Autodesk Inventor part; units mm, degrees
ref_plane "YZ Plane" through (0, 0, 0) normal (1, 0, 0) x (0, 1, 0)
ref_plane "XZ Plane" through (0, 0, 0) normal (0, 1, 0) x (-1, 0, 0)
ref_plane "XY Plane" through (0, 0, 0) normal (0, 0, 1) x (1, 0, 0)
ref_plane "Work Plane1" through (1.1136, 1.5, 0.2896) normal (0, -1, 0) x (1, 0, 0)
sketch "Sketch3" plane through (1.1136, 1.5, 0.2896) normal (0, -1, 0) x (1, 0, 0)
  line L0 (-8.5, 0) -> (-8.5, 5) construction
  line L1 (-8.5, 5) -> (-1.5, 5) construction
  line L2 (-1.5, 5) -> (-1.5, 0) construction
  line L3 (0, 0) -> (-1.5, 0) construction
  line L4 (0, 0) -> (0, 6) construction
  line L5 (0, 6) -> (-22.065, 6) construction
  line L6 (-22.065, 0) -> (-22.065, 6) construction
  line L7 (-20.565, 0) -> (-22.065, 0) construction
  line L8 (-20.565, 0) -> (-20.565, 5) construction
  line L9 (-20.565, 5) -> (-13.565, 5) construction
  line L10 (-13.565, 5) -> (-13.565, 0) construction
  line L11 (-8.5, 0) -> (-13.565, 0) construction
  line L12 (-0.8, 0) -> (-21.265, 0)
  line L13 (-21.265, 0) -> (-21.265, 5.3)
  line L14 (-21.265, 5.3) -> (-0.8, 5.3)
  line L15 (-0.8, 5.3) -> (-0.8, 0)
  point P0 (-1.1136, -0.2896)
  dimension "d26" = 0.8
  dimension "d27" = 0.8
  dimension "d28" = 0.7
extrude "Extrusion3" add sketch "Sketch3" along normal blind 3
sketch "Sketch4" plane through (1.1136, 1.5, 0.2896) normal (0, 1, 0) x (1, 0, 0)
  line L0 (-8.5, 0) -> (-8.5, -5) construction
  line L1 (-8.5, -5) -> (-1.5, -5) construction
  line L2 (-1.5, -5) -> (-1.5, 0) construction
  line L3 (0, 0) -> (-1.5, 0) construction
  line L4 (0, 0) -> (0, -6) construction
  line L5 (0, -6) -> (-22.065, -6) construction
  line L6 (-22.065, 0) -> (-22.065, -6) construction
  line L7 (-20.565, 0) -> (-22.065, 0) construction
  line L8 (-20.565, 0) -> (-20.565, -5) construction
  line L9 (-20.565, -5) -> (-13.565, -5) construction
  line L10 (-13.565, -5) -> (-13.565, 0) construction
  line L11 (-8.5, 0) -> (-13.565, 0) construction
  line L12 (-2, 0) -> (-8, 0)
  line L13 (-8, 0) -> (-8, -4.3)
  line L14 (-8, -4.3) -> (-2, -4.3)
  line L15 (-2, -4.3) -> (-2, 0)
  line L16 (-0.8, 0) -> (-21.265, 0)
  line L17 (-14.065, 0) -> (-20.065, 0)
  line L18 (-20.065, 0) -> (-20.065, -4.3)
  line L19 (-20.065, -4.3) -> (-14.065, -4.3)
  line L20 (-14.065, -4.3) -> (-14.065, 0)
  point P0 (-1.1136, 0.2896)
  point P1 (-5, 0)
  point P2 (-11.0325, 0)
  dimension "d31" = 0.5
  dimension "d32" = 0.5
  dimension "d33" = 0.7
  dimension "d34" = 0.7
  dimension "d35" = 0.5
  dimension "d36" = 0.5
extrude "Extrusion4" add sketch "Sketch4" along normal blind 7
fillet "Fillet6" radius 1 4 edges at (-20.1514, 0, 5.5896) (-20.1514, 0, 0.2896) (0.3136, 0, 5.5896) (0.3136, 0, 0.2896)
fillet "Fillet6" radius 1 4 edges at (-3.8864, 8.5, 4.5896) (-3.8864, 8.5, 0.2896) (-15.9514, 8.5, 0.2896) (-15.9514, 8.5, 4.5896)
properties part number "Holster_Button"
Source: CAD feature listing. Evaluate the final solid. Frame: model axes, mm. A direction names the side the tool comes from. Round coordinates to 2 decimals unless told otherwise and drop trailing zeros. Loops run counter-clockwise (first coordinate to the right, second up) from the corner with the lowest first, then second, coordinate; pieces in that order, holes last. Notation, with made-up numbers: M 81,-31 L 100,-31 A11 cw 100,-21 Z; hole C 13,66.5 d4. An arc over 180 degrees is marked long. Use a Markdown table: item, result. Add a question column.
1. Cut plane C-C, the plane x = -1.25. Output: boundary loops of the cut face in (y, z).
2. Set-up query: faces 1 (the flat face through (-0.886, 5, 2)), 2 (the flat face through (-12.951, 5, 2)), 3 (the flat face through (-16, 4, 4.59)). Return all of +Z, -Z, +X, -X, +Y, -Y with unobstructed straight access to the full face (end or side cutting, diameter ignored); none if empty.
3. Cut plane D-D, the plane z = 4.15. Output: boundary loops of the cut face in (x, y).
4. Cut plane B-B, the plane z = 3.3. Output: boundary loops of the cut face in (x, y), and give its area (3 significant figures).
5. Ray query, line 1 along X through (y, z) = (7.25, 2.7); line 2 along Y through (x, z) = (-18.25, 4.9); line 3 along Z through (x, y) = (-2.5, 3). Return the intervals inside material, ascending. Write a range as [from, to].
6. Contact query for flat-ended pins moving along their axis: pin 1 (2 mm diameter, centred on y = 4, z = 1.5, fed in from -X); pin 2 (1.8 mm diameter, centred on x = -15, y = 4.5, fed in from +Z); pin 3 (2 mm diameter, centred on y = 4.5, z = 1.5, fed in from +X). Output: stop coordinate, or through.
7. Cut plane A-A, the plane y = 4.5. Output: boundary loops of the cut face in (x, z).
Solution:
| question | item | result |
|---|---|---|
| 1 | outline | M -1.5,0.29 L 7.5,0.29 A1 ccw 8.5,1.29 L 8.5,3.59 A1 ccw 7.5,4.59 L 1.5,4.59 L 1.5,5.59 L -1.5,5.59 Z |
| 2 | face 1 | +Z, -Z, +X, +Y |
| 2 | face 2 | +Z, -Z, +Y |
| 2 | face 3 | +Z, +X, -X, +Y |
| 3 | outline | M -20.15,-1.5 L 0.31,-1.5 L 0.31,1.5 L -0.89,1.5 L -0.89,8.33 L -6.89,8.33 L -6.89,1.5 L -12.95,1.5 L -12.95,8.33 L -18.95,8.33 L -18.95,1.5 L -20.15,1.5 Z |
| 4 | outline | M -20.15,-1.5 L 0.31,-1.5 L 0.31,1.5 L -0.89,1.5 L -0.89,8.5 L -6.89,8.5 L -6.89,1.5 L -12.95,1.5 L -12.95,8.5 L -18.95,8.5 L -18.95,1.5 L -20.15,1.5 Z |
| 4 | area | 145 mm2 |
| 5 | line 1 | x = [-18.95, -12.95], [-6.89, -0.89] |
| 5 | line 2 | y = [-1.5, 1.5] |
| 5 | line 3 | z = [0.29, 4.59] |
| 6 | pin 1 | stops at x = -18.95 |
| 6 | pin 2 | stops at z = 4.59 |
| 6 | pin 3 | stops at x = -0.89 |
| 7 | outline | M -18.95,0.29 L -12.95,0.29 L -12.95,4.59 L -18.95,4.59 Z; M -6.89,0.29 L -0.89,0.29 L -0.89,4.59 L -6.89,4.59 Z |
